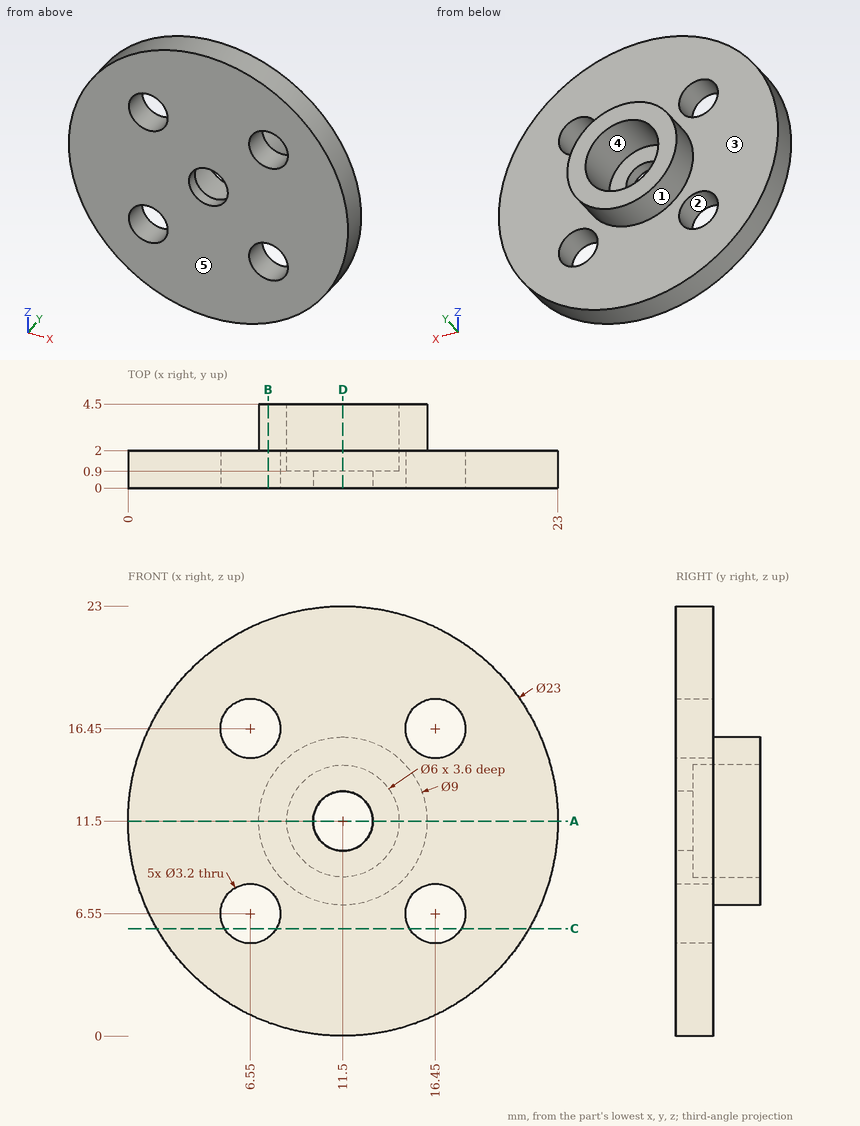
Here's the drawing with two shaded views (mm, measured from the low corner). I have some questions. A direction names the side the tool comes from. Round coordinates to 2 decimals unless told otherwise and drop trailing zeros. Order: outer loops, then holes, each group sorted by start corner. A loop starts at its lowest first (then second) coordinate and runs counter-clockwise, first axis right, second up. Notation, with made-up numbers: (21.5, 29) -> (30.5, 29) arc R10 ccw to (30.5, 33) -> close; hole circle Ø8 at (22, -27). An arc over 180 degrees is marked (long way). Return JSON: item names as keys, results as strings.
Q1. For pin 1 Ø3.5 at (x, z) = (6.55, 16.45) entering from +Y; pin 2 Ø3.5 at (x, z) = (11.5, 11.5) entering from +Y; pin 3 Ø2 at (x, y) = (7, 0.5) entering from +Z, each with a flat end and sliding along its axis, tell me the tip position at first contact or that it passes through.
Filled sheet:
{"pin 1": "stops at y = 2", "pin 2": "stops at y = 0.9", "pin 3": "stops at z = 22.45"}
Q2. I need wall thicknesses on line 1 along Z through (x, y) = (15, 0.35) (1 decimal); line 2 along X through (y, z) = (1.8, 7.25) (1 decimal); line 3 along X through (y, z) = (0.55, 11.5). Which ranges of each line are inside material? Lowest first, please. Write a range as from..to.
Filled sheet:
{"line 1": "z = 0.5..5.9, 7.2..15.8, 17.1..22.5", "line 2": "x = 0.8..5.1, 8..15, 17.9..22.2", "line 3": "x = 0..9.9, 13.1..23"}
Q3. If we mould it in two halves opening along X, with no side actions, what happens to the marked faces 1, 2 and 3? For each: released by +X, released by -X, zero draft, split by the parting line, or undercut.
Filled sheet:
{"face 1": "split by the parting line", "face 2": "undercut", "face 3": "zero draft"}
Q4. If we section it at B-B on x = 7.5: List the corners of the cut face in (y, z) for me.
Filled sheet:
{"outline": "(0, 0.72) -> (2, 0.72) -> (2, 5.26) -> (0, 5.26) -> close; (0, 7.84) -> (2, 7.84) -> (2, 9.44) -> (4.5, 9.44) -> (4.5, 13.56) -> (2, 13.56) -> (2, 15.16) -> (0, 15.16) -> close; (0, 17.74) -> (2, 17.74) -> (2, 22.28) -> (0, 22.28) -> close"}
Q5. If we section it at D-D on x = 11.5: List the corners of the cut face in (y, z) for me.
Filled sheet:
{"outline": "(0, 0) -> (2, 0) -> (2, 7) -> (4.5, 7) -> (4.5, 8.5) -> (0.9, 8.5) -> (0.9, 9.9) -> (0, 9.9) -> close; (0, 13.1) -> (0.9, 13.1) -> (0.9, 14.5) -> (4.5, 14.5) -> (4.5, 16) -> (2, 16) -> (2, 23) -> (0, 23) -> close"}
Q6. If we section it at A-A on z = 11.5: List the corners of the cut face in (x, y) for me, plus the area to 3 significant figures.
Filled sheet:
{"outline": "(0, 0) -> (9.9, 0) -> (9.9, 0.9) -> (8.5, 0.9) -> (8.5, 4.5) -> (7, 4.5) -> (7, 2) -> (0, 2) -> close; (13.1, 0) -> (23, 0) -> (23, 2) -> (16, 2) -> (16, 4.5) -> (14.5, 4.5) -> (14.5, 0.9) -> (13.1, 0.9) -> close", "area": "44.0 mm^2"}
Q7. Which directions (+Z, -Z, +X, -X, +Y, -Y) give clear straight access to the entire face, cutting with the end or side of a thin tool? Please do the marked faces 4 and 5.
Filled sheet:
{"face 4": "+Y", "face 5": "+Z, -Z, +X, -X, -Y"}
Q8. If we section it at C-C on z = 5.75: List the corners of the cut face in (x, y) for me (1 decimal).
Filled sheet:
{"outline": "(1.5, 0) -> (5.2, 0) -> (5.2, 2) -> (1.5, 2) -> close; (7.9, 0) -> (15.1, 0) -> (15.1, 2) -> (7.9, 2) -> close; (17.8, 0) -> (21.5, 0) -> (21.5, 2) -> (17.8, 2) -> close"}
